Check sheet for the drawn part. Datum: minimum x, y, z corner. Units: mm. Round coordinates to 2 decimals unless told otherwise and drop trailing zeros. Order: outer loops, then holes, each group sorted by start corner. A loop starts at its lowest first (then second) coordinate and runs counter-clockwise, first axis right, second up. Notation, with made-up numbers: M 66,52.5 L 117,52.5 A10 ccw 117,66.5 Z; hole C 79,45 d7. An arc over 180 degrees is marked long. Use one line per item in the form item = value. Start each with the question number.
Item 1: Cross-section at D-D on z = 16.75. Enter the section's corners in (x, y) (3 decimals), then the cut area to 3 significant figures.
Item 2: Cross-section at A-A on y = 1.75. Enter the section's corners in (x, z).
Item 3: Cross-section at B-B on x = 192. Enter the section's corners in (y, z) (3 decimals), then the cut area to 3 significant figures.
Item 4: Go/stop test with a flat-tipped pin: pin 1 Ø1 at (y, z) = (2, 7) entering from +X. Record where the tip stops, or that it passes through.
Item 5: Cross-section at C-C on z = 2. Enter the section's corners in (x, y) (3 decimals).
Item 6: Thickness scan on probe 1 along X at (y, z) = (0.65, 12.25); probe 2 along X at (y, z) = (1, 11); probe 3 along Z at (x, y) = (192, 2.15). Record the ranges inside material, lowest first. Write a range as [from, to].
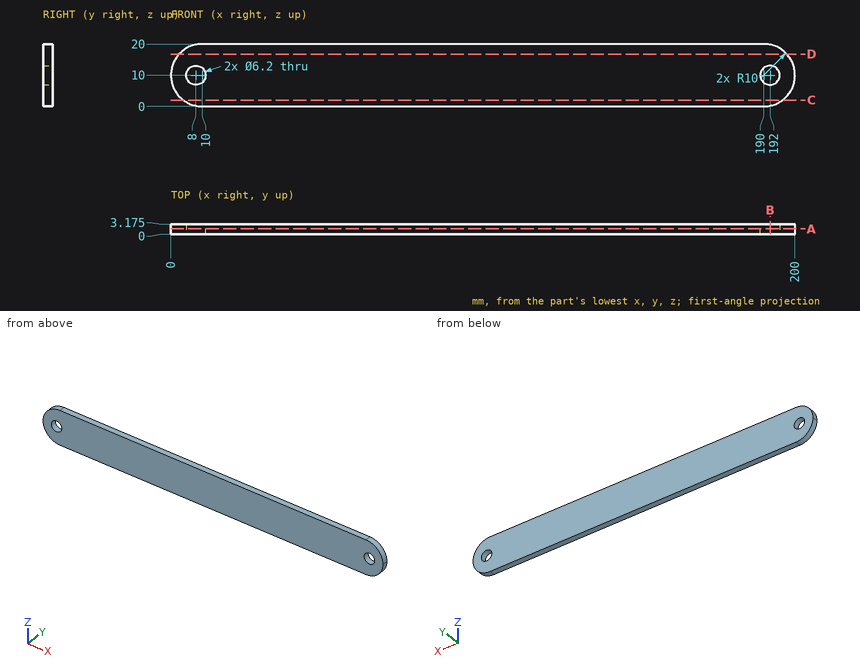
Output values:
q1.outline = M 2.622,0 L 197.378,0 L 197.378,3.175 L 2.622,3.175 Z
q1.area = 618 mm2
q2.outline = M 0,10 A10 ccw 10,0 L 190,0 A10 ccw 200,10 A10 ccw 190,20 L 10,20 A10 ccw Z; hole C 8,10 d6.2; hole C 192,10 d6.2
q3.outline = M 0,0.202 L 3.175,0.202 L 3.175,6.9 L 0,6.9 Z; M 0,13.1 L 3.175,13.1 L 3.175,19.798 L 0,19.798 Z
q3.area = 42.5 mm2
q4.pin_1 = 199.68
q5.outline = M 4,0 L 196,0 L 196,3.175 L 4,3.175 Z
q6.probe_1 = [0.26, 5.87], [10.13, 189.87], [194.13, 199.74]
q6.probe_2 = [0.05, 5.07], [10.93, 189.07], [194.93, 199.95]
q6.probe_3 = [0.2, 6.9], [13.1, 19.8]
